```python
from build123d import *

# Parameters (mm, degrees)
F0_W     = 150
F0_H     = 45.5
F1_DEPTH = 35
F2_W     = 150
F2_H     = 35.5
F3_DEPTH = 25
F4_R     = 12.75
F5_DEPTH = 8.5
F6_D     = 6.5
F6_DEPTH = 5
F6_TIP   = 1.9527970118


with BuildPart() as f1:
    # F0 (on Top) → F1 (new body)
    with BuildSketch(Plane.XY):
        Rectangle(F0_W, F0_H)
    extrude(amount=F1_DEPTH)

    # F2 (on face) → F3 (cut)
    with BuildSketch(Plane.XY.offset(35)):
        Rectangle(F2_W, F2_H)
    extrude(amount=-F3_DEPTH, mode=Mode.SUBTRACT)

    # F4 (on face) → F5 (cut)
    with BuildSketch(Plane.XY.offset(10)):
        Circle(F4_R)
    extrude(amount=-F5_DEPTH, mode=Mode.SUBTRACT)

    # F6
    with Locations(Plane.XY.offset(10)):
        with Locations((55, 0), (-55, 0)):
            Hole(F6_D / 2, depth=F6_DEPTH)
            with Locations((0, 0, -(F6_DEPTH + F6_TIP / 2))):  # 118° drill point
                Cone(0, F6_D / 2, F6_TIP, mode=Mode.SUBTRACT)


solid = f1.part
```
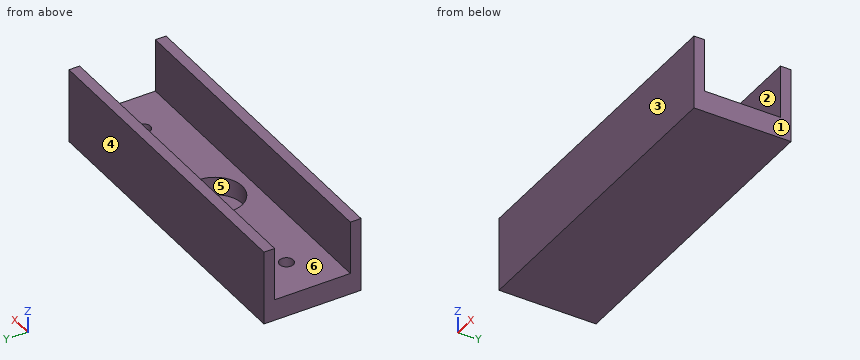
Source: CAD feature listing. Evaluate the final solid. Frame: model axes, mm. Face numbers are marked on the shaded views. A direction names the side the tool comes from. Round coordinates to 2 decimals unless told otherwise and drop trailing zeros. Loops run counter-clockwise (first coordinate to the right, second up) from the corner with the lowest first, then second, coordinate; pieces in that order, holes last. Notation, with made-up numbers: M 60.5,-31.5 L 108.5,-31.5 A11 cw 108.5,-15.5 Z; hole C 25,29.25 d3. An arc over 180 degrees is marked long. Put each result on its own line as item: value.
(1) Section C-C, the plane z = 20. Return loops of the section in (x, y), and give its area (3 significant figures).
Solutions:
outline: M -75,-22.75 L 75,-22.75 L 75,-17.75 L -75,-17.75 Z; M -75,17.75 L 75,17.75 L 75,22.75 L -75,22.75 Z
area: 1,500 mm²
(2) First-contact query: pin 1 (8.5 mm diameter, centred on x = -55, y = 0, fed in from +Z); pin 2 (10.5 mm diameter, centred on x = 6, y = -1, fed in from +Z). Flat tips, straight axial feed; report the tip coordinate or a pass-through.
Solutions:
pin 1: z = 10
pin 2: z = 1.5
(3) Section A-A, the plane z = 7.5. Return loops of the section in (x, y), and give its area (3 significant figures).
Solutions:
outline: M -75,-22.75 L 75,-22.75 L 75,22.75 L -75,22.75 Z; hole C -55,0 d6.5; hole C 0,0 d25.5; hole C 55,0 d6.5
area: 6,250 mm²
(4) Access query for the marked faces 4, 5 and 6. Directions: +Z, -Z, +X, -X, +Y, -Y. A direction counts if a zero-diameter tool reaches every point of the face in a straight line with its end or side. Return the directions, or none.
Solutions:
face 4: +Z, -Z, +X, -X, +Y
face 5: +Z
face 6: +Z, +X, -X
(5) Ray query, line 1 (Y direction, x = 0, z = 5); line 2 (Y direction, x = 41.5, z = 31); line 3 (Z direction, x = -5.5, y = -2.5). Return the intervals inside material, ascending. Write a range as [from, to].
Solutions:
line 1: [-22.75, -12.75], [12.75, 22.75]
line 2: [-22.75, -17.75], [17.75, 22.75]
line 3: [0, 1.5]
(6) Section D-D, the plane y = -6. Return loops of the section in (x, z).
Solutions:
outline: M -75,0 L 75,0 L 75,10 L 11.25,10 L 11.25,1.5 L -11.25,1.5 L -11.25,10 L -75,10 Z
(7) Pull-direction query (Y, two-part tool) for the marked faces 1, 2 and 3; classes: released by +Y, released by -Y, zero draft, split by the parting line, or undercut.
Solutions:
face 1: zero draft
face 2: undercut
face 3: released by -Y
(8) Section B-B, the plane x = 19. Return loops of the section in (y, z), and give its area (3 significant figures).
Solutions:
outline: M -22.75,0 L 22.75,0 L 22.75,35 L 17.75,35 L 17.75,10 L -17.75,10 L -17.75,35 L -22.75,35 Z
area: 705 mm²
